from build123d import *

# Parameters (mm, degrees)
SKETCH1_R           = 12.5
BOSS_EXTRUDE1_DEPTH = 5
CUT_EXTRUDE2_REACH  = 20.371
SKETCH3_R           = 3
CUT_EXTRUDE3_REACH  = 20.371
SKETCH4_R           = 1.525


with BuildPart() as part:
    # Sketch1 → Boss-Extrude1 (new body)
    with BuildSketch(Plane.XY):
        Circle(SKETCH1_R)
    extrude(amount=BOSS_EXTRUDE1_DEPTH)

    # Sketch3 → Cut-Extrude2 (cut, up to next)
    with BuildSketch(Plane.XY.offset(5), mode=Mode.PRIVATE) as cut_extrude2_sk1:
        Circle(SKETCH3_R)
    cut_extrude2_tool1 = extrude(cut_extrude2_sk1.sketch, amount=-CUT_EXTRUDE2_REACH, mode=Mode.PRIVATE) & part.part
    add(cut_extrude2_tool1.solids().sort_by_distance((0, 0, 5))[0], mode=Mode.SUBTRACT)

    # Sketch4 → Cut-Extrude3 (cut, up to next)
    with BuildSketch(Plane.XY.offset(5), mode=Mode.PRIVATE) as cut_extrude3_sk1:
        with Locations((0, 9)):
            Circle(SKETCH4_R)
    cut_extrude3_tool1 = extrude(cut_extrude3_sk1.sketch, amount=-CUT_EXTRUDE3_REACH, mode=Mode.PRIVATE) & part.part
    # Sketch4 → Cut-Extrude3 (cut, up to next)
    with BuildSketch(Plane.XY.offset(5), mode=Mode.PRIVATE) as cut_extrude3_sk2:
        with Locations((7.794228634, -4.5)):
            Circle(SKETCH4_R)
    cut_extrude3_tool2 = extrude(cut_extrude3_sk2.sketch, amount=-CUT_EXTRUDE3_REACH, mode=Mode.PRIVATE) & part.part
    # Sketch4 → Cut-Extrude3 (cut, up to next)
    with BuildSketch(Plane.XY.offset(5), mode=Mode.PRIVATE) as cut_extrude3_sk3:
        with Locations((-7.794228634, -4.5)):
            Circle(SKETCH4_R)
    cut_extrude3_tool3 = extrude(cut_extrude3_sk3.sketch, amount=-CUT_EXTRUDE3_REACH, mode=Mode.PRIVATE) & part.part
    add(cut_extrude3_tool1.solids().sort_by_distance((0, 9, 5))[0], mode=Mode.SUBTRACT)
    add(cut_extrude3_tool2.solids().sort_by_distance((7.794229, -4.5, 5))[0], mode=Mode.SUBTRACT)
    add(cut_extrude3_tool3.solids().sort_by_distance((-7.794229, -4.5, 5))[0], mode=Mode.SUBTRACT)


solid = part.part
Model file for the job. Use its own axes, mm. Round coordinates to 2 decimals unless told otherwise and drop trailing zeros. Loops run counter-clockwise (first coordinate to the right, second up) from the corner with the lowest first, then second, coordinate; pieces in that order, holes last. Notation, with made-up numbers: M 89,-14 L 146,-14 A8 ccw 146,-10 Z; hole C 49,-26.75 d9. An arc over 180 degrees is marked long. One line per question, with ' | ' between items.
1) Band-saw the part on D-D (x = 7.5). Give the cut face in (y, z), then the cut area to 3 significant figures.
Solved:
outline: M -10,0 L -6,0 L -6,5 L -10,5 Z; M -3,0 L 10,0 L 10,5 L -3,5 Z | area: 85.0 mm²
2) Drill centre lines: line 1 along Y through (x, z) = (0, 2.5) (3 decimals); line 2 along X through (y, z) = (-5, 2.9); line 3 along Y through (x, z) = (1, 2.3). Where is each one in solid material? Low to high.
Solved:
line 1: y = -12.5 to -3, 3 to 7.475, 10.525 to 12.5 | line 2: x = -11.46 to -9.23, -6.35 to 6.35, 9.23 to 11.46 | line 3: y = -12.46 to -2.83, 2.83 to 7.85, 10.15 to 12.46
3) Band-saw the part on B-B (z = 0.5). Give the cut face in (x, y) (3 decimals).
Solved:
outline: C 0,0 d25; hole C -7.794,-4.5 d3.05; hole C 0,0 d6; hole C 0,9 d3.05; hole C 7.794,-4.5 d3.05
4) Mould opens along Y. For faces 1 (the cylindrical face through (-3, 0, 3)), 2 (the flat face through (3, -3, 5)), 3 (the cylindrical face through (11.923, 3.755, 2.465)) say: +Y half, -Y half, draft (parallel to the pull), parting line (faces both ways), or undercut.
Solved:
face 1: undercut | face 2: draft | face 3: parting line
5) Flat gauge pins, fed straight in: pin 1 (2.5 mm diameter, centred on x = 7.79, y = -4.5, fed in from -Z); pin 2 (2 mm diameter, centred on x = 9.5, z = 4, fed in from -Y). Where does each tip first touch, or does it go through?
Solved:
pin 1: passes through | pin 2: stops at y = -9.17
6) Band-saw the part on A-A (x = 0). Give the cut face in (y, z) (3 decimals), then the cut area to 4 significant figures.
Solved:
outline: M -12.5,0 L -3,0 L -3,5 L -12.5,5 Z; M 3,0 L 7.475,0 L 7.475,5 L 3,5 Z; M 10.525,0 L 12.5,0 L 12.5,5 L 10.525,5 Z | area: 79.75 mm²
7) Band-saw the part on C-C (y = 9). Give the cut face in (x, z) (3 decimals), then the cut area to 3 significant figures.
Solved:
outline: M -8.675,0 L -1.525,0 L -1.525,5 L -8.675,5 Z; M 1.525,0 L 8.675,0 L 8.675,5 L 1.525,5 Z | area: 71.5 mm²
